The model under review builds one solid part; all positions refer to its coordinate system, in mm. A direction names the side the tool comes from. Give positions to 0.01 mm unless a question says otherwise; leave off trailing zeros. Loops run counter-clockwise (first coordinate to the right, second up) from the corner with the lowest first, then second, coordinate; pieces in that order, holes last. Notation, with made-up numbers: M 28,6.5 L 85,6.5 A36 cw 85,44.5 Z; hole C 76.5,22.5 d8. An arc over 180 degrees is marked long. One line per item, written item: value. Start each with the question number.
Q1. For faces 1 (the face through (0.45, 33.99, 1.43)), 2 (the face through (0, 0, 0)), list the 3-axis set-ups (+Z, -Z, +X, -X, +Y, -Y) from which the entire face can be reached by the end or side of a thin tool; tool diameter is ignored.
Q2. We need section C-C on z = 1.15. Write out the cut boundary in (x, y).
Q3. For pin 1 (1.5 mm diameter, centred on x = -2, y = 32.5, fed in from -Z), flat-tipped, find the tip position at first contact; note if it passes through.
Q4. We need section B-B on y = 21. Write out the cut boundary in (x, z).
Q5. To check wall thickness, follow line 1 along Y through (x, z) = (0.9, 1.8); line 2 along Z through (x, y) = (-2.2, 9); line 3 along X through (y, z) = (10.5, -0.85). State the ranges of each line that lie inside material, in increasing order. Write a range as from..to.
Q6. We need section A-A on x = 0. Write out the cut boundary in (y, z).
Q7. We need section D-D on x = 2.25. Write out the cut boundary in (y, z), plus the area to 3 significant figures.
```python
from build123d import *

# Parameters (mm, degrees)
BOSS_EXTRUDE1_DEPTH = 30
SKETCH5_R           = 1.5
BOSS_EXTRUDE2_DEPTH = 8.091605471
SKETCH5_2_R         = 1.5
BOSS_EXTRUDE3_DEPTH = 8


with BuildPart() as part:
    # Sketch3 → Boss-Extrude1 (new body)
    with BuildSketch(Plane(origin=(0, 0, 0), x_dir=(1, 0, 0), z_dir=(0, 1, 0))):
        Polygon((-2.886751346, 0), (-1.443375673, -2.5), (1.443375673, -2.5), (2.886751346, 0), (1.443375673, 2.5), (-1.443375673, 2.5), align=None)
    extrude(amount=BOSS_EXTRUDE1_DEPTH)

    # Sketch5 → Boss-Extrude2 (add)
    with BuildSketch(Plane(origin=(0, 30, 0), x_dir=(1, 0, 0), z_dir=(0, 1, 0))):
        with Locations(Location((0, 0, 0), (0, 0, 270))):
            Circle(SKETCH5_R)
    extrude(amount=BOSS_EXTRUDE2_DEPTH)

    # Sketch5_2 → Boss-Extrude3 (add)
    with BuildSketch(Plane(origin=(0, 30, 0), x_dir=(1, 0, 0), z_dir=(0, 1, 0))):
        with Locations(Location((0, 0, 0), (0, 0, 270))):
            Circle(SKETCH5_2_R)
    extrude(amount=BOSS_EXTRUDE3_DEPTH)


solid = part.part
```
Solved:
1. face 1: +Y
1. face 2: +Z, -Z, +X, -X, -Y
2. outline: M -2.22,0 L 2.22,0 L 2.22,30 L 0.96,30 L 0.96,38.09 L -0.96,38.09 L -0.96,30 L -2.22,30 Z
3. pin 1: z = -0.83
4. outline: M -2.89,0 L -1.44,-2.5 L 1.44,-2.5 L 2.89,0 L 1.44,2.5 L -1.44,2.5 Z
5. line 1: 0..30
5. line 2: -1.19..1.19
5. line 3: -2.4..2.4
6. outline: M 0,-2.5 L 30,-2.5 L 30,-1.5 L 38.09,-1.5 L 38.09,1.5 L 30,1.5 L 30,2.5 L 0,2.5 Z
7. outline: M 0,-1.1 L 30,-1.1 L 30,1.1 L 0,1.1 Z
7. area: 66.2 mm2
